```python
from build123d import *

# Parameters (mm, degrees)
BOSS_EXTRUDE1_DEPTH = 5
CIRPATTERN1_COUNT   = 3
CIRPATTERN1_ANGLE   = 120
SKETCH2_R           = 2.5
CUT_EXTRUDE1_DEPTH  = 99.777078193
CIRPATTERN2_COUNT   = 6


with BuildPart() as part:
    # Sketch1 → Boss-Extrude1 (new body)
    with BuildSketch(Plane(origin=(0, 0, 0), x_dir=(1, 0, 0), z_dir=(0, 1, 0))):
        with BuildLine():
            ThreePointArc((-15.9, 47.404535648), (-50, 0), (-15.9, -47.404535648))
            Line((-15.9, -47.404535648), (-15.9, 47.404535648))
        make_face()
        with BuildLine():
            ThreePointArc((-15.9, -47.404535648), (0, -50), (15.9, -47.404535648))
            Line((15.9, -47.404535648), (15.9, 47.404535648))
            ThreePointArc((15.9, 47.404535648), (0, 50), (-15.9, 47.404535648))
            Line((-15.9, 47.404535648), (-15.9, -47.404535648))
        make_face()
        with BuildLine():
            Line((-15.9, -70.5), (15.9, -70.5))
            Line((15.9, -70.5), (15.9, -47.404535648))
            ThreePointArc((15.9, -47.404535648), (0, -50), (-15.9, -47.404535648))
            Line((-15.9, -47.404535648), (-15.9, -70.5))
        make_face()
        with BuildLine():
            ThreePointArc((-15.9, 47.404535648), (0, 50), (15.9, 47.404535648))
            Line((15.9, 47.404535648), (15.9, 70.5))
            Line((15.9, 70.5), (-15.9, 70.5))
            Line((-15.9, 70.5), (-15.9, 47.404535648))
        make_face()
        with BuildLine():
            Line((15.9, 47.404535648), (15.9, -47.404535648))
            ThreePointArc((15.9, -47.404535648), (40.589407485, -29.197602641), (50, 0))
            ThreePointArc((50, 0), (40.589407485, 29.197602641), (15.9, 47.404535648))
        make_face()
    boss_extrude1 = extrude(amount=BOSS_EXTRUDE1_DEPTH)

    # CirPattern1: Boss-Extrude1 ×3 about axis
    cirpattern1_axis = Axis((0, 0, 0), (0, 1, 0))
    for i in range(1, CIRPATTERN1_COUNT):
        add(boss_extrude1.rotate(cirpattern1_axis, i * CIRPATTERN1_ANGLE / (CIRPATTERN1_COUNT - 1)))

    # Sketch2 → Cut-Extrude1 (cut, through all)
    with BuildSketch(Plane(origin=(0, 5, 0), x_dir=(1, 0, 0), z_dir=(0, 1, 0))):
        with Locations(Location((49.376524227, -34.477351338, 0), (0, 0, 270))):
            Circle(SKETCH2_R)
    cut_extrude1 = extrude(amount=-CUT_EXTRUDE1_DEPTH, mode=Mode.SUBTRACT)

    # CirPattern2: Cut-Extrude1 ×6 about axis
    cirpattern2_axis = Axis((0, 0, 0), (0, 1, 0))
    for i in range(1, CIRPATTERN2_COUNT):
        add(cut_extrude1.rotate(cirpattern2_axis, i * 360 / CIRPATTERN2_COUNT), mode=Mode.SUBTRACT)


solid = part.part
```
Check sheet for the modelled part. Datum: model origin and axes. Units: mm. A direction names the side the tool comes from. Give positions to 0.01 mm unless a question says otherwise; leave off trailing zeros. Write each loop counter-clockwise with the first axis right and the second up, starting at its lowest first coordinate (ties: lowest second). Pieces come first, ordered by that corner, then holes. Notation, with made-up numbers: (88.5, 51) -> (134.5, 51) arc R15 cw to (134.5, 66) -> close; hole circle Ø3 at (5.25, 52.25). An arc over 180 degrees is marked (long way). Use CSV: the item, a comma, the result in double quotes. Start each with the question number.
Q1. Release check for a two-part mould opening along X. For faces 4 (the flat face through (43.2, 2.5, -43.3)), 5 (the cylindrical face through (-55.504, 2.535, 27.832)), 6 (the flat face through (-61.166, 2.465, 35.057)), 7 (the flat face through (0, 2, -70.5)) record: +X half, -X half, draft (parallel to the pull), parting line (faces both ways), or undercut.
Q2. Scan lines: line 1 along X through (y, z) = (0.6, 60); line 2 along X through (y, z) = (1.6, 10.5); line 3 along X through (y, z) = (4, -43.5). Record each from-to range of solid material in increasing order.
Q3. Tool access check on faces 1 (the cylindrical face through (-24.88, 2.46, -43.37)), 2 (the flat face through (-58.864, 2.465, 15.625)), 3 (the flat face through (-43.2, 2.5, 43.3)). Record the directions out of +Z, -Z, +X, -X, +Y, -Y that give a thin tool (end or side, any length) a straight path to the whole face; none if there is none.
Q4. Cross-section at C-C on y = 1.45. Count the separate pieces of the cut face and the enclosed holes in it, and give its area (3 significant figures).
Q5. Cross-section at A-A on x = 5.17. Enter the section's corners in (y, z), and give its area (3 significant figures).
Q6. Cross-section at B-B on z = -42.5. Enter the section's corners in (x, y), and give its area (3 significant figures).
Q7. Cross-section at D-D on z = 54. Enter the section's corners in (x, y), and give its area (3 significant figures).
Q8. Depth check by flat-ended pin: P1, Ø3, axis at x = -44, z = 21, coming from the -Y side; P2, Ø2.5, axis at y = 3, z = -57.5, coming from the -X side; P3, Ø1.5, axis at y = 2, z = 59, coming from the +X side. Enter the tip coordinate at first touch or a pass-through.
Working result:
1,face 4,"undercut"
1,face 5,"undercut"
1,face 6,"-X half"
1,face 7,"draft"
2,line 1,"x = -15.9 to -7.67, -2.67 to 15.9"
2,line 2,"x = -49.99 to 49.99"
2,line 3,"x = -56.29 to -43.54, -24.65 to 24.65, 43.54 to 56.29"
3,face 1,"-Z, +Y, -Y"
3,face 2,"-X, +Y, -Y"
3,face 3,"+Z, +Y, -Y"
4,separate pieces,"1"
4,enclosed holes,"6"
4,area,"11,800 mm^2"
5,outline,"(0, -70.5) -> (5, -70.5) -> (5, -62.5) -> (0, -62.5) -> close; (0, -57.5) -> (5, -57.5) -> (5, 70.5) -> (0, 70.5) -> close"
5,area,"680 mm^2"
6,outline,"(-56.87, 0) -> (-41.81, 0) -> (-41.81, 5) -> (-56.87, 5) -> close; (-26.34, 0) -> (26.34, 0) -> (26.34, 5) -> (-26.34, 5) -> close; (41.81, 0) -> (56.87, 0) -> (56.87, 5) -> (41.81, 5) -> close"
6,area,"414 mm^2"
7,outline,"(-15.9, 0) -> (15.9, 0) -> (15.9, 5) -> (-15.9, 5) -> close"
7,area,"159 mm^2"
8,P1,"stops at y = 0"
8,P2,"stops at x = -15.9"
8,P3,"stops at x = 15.9"
